Source: CAD feature listing. Evaluate the final solid. Frame: model axes, mm. Face numbers are marked on the shaded views. Give positions to 0.01 mm unless a question says otherwise; leave off trailing zeros. Order: outer loops, then holes, each group sorted by start corner. A loop starts at its lowest first (then second) coordinate and runs counter-clockwise, first axis right, second up.
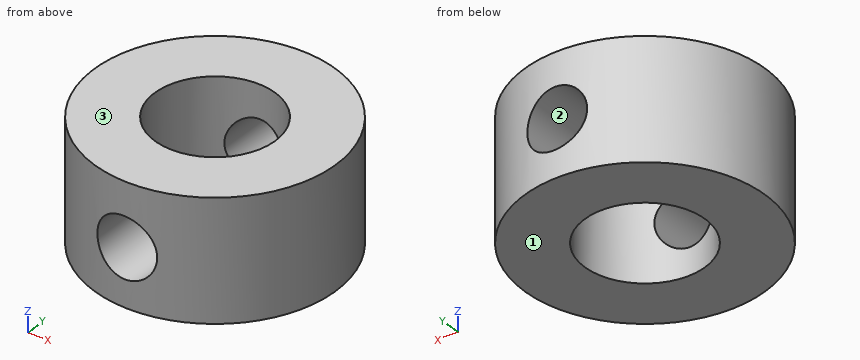
from build123d import *

# Parameters (mm, degrees)
F0_R     = 10
F1_DEPTH = 10
F2_R     = 5
F3_DEPTH = 25
F4_R     = 2.5
F5_DEPTH = 12.5


with BuildPart() as f1:
    # F0 (on Top) → F1 (new body)
    with BuildSketch(Plane.XY):
        Circle(F0_R)
    extrude(amount=F1_DEPTH)

    # F2 (on face) → F3 (cut)
    with BuildSketch(Plane.XY.offset(10)):
        Circle(F2_R)
    extrude(amount=-F3_DEPTH, mode=Mode.SUBTRACT)

    # F4 (on Front) → F5 (cut, symmetric)
    with BuildSketch(Plane.XZ):
        with Locations((0, 4.75)):
            Circle(F4_R)
    extrude(amount=F5_DEPTH, both=True, mode=Mode.SUBTRACT)


solid = f1.part
(1) Section B-B, the plane y = 0. Return loops of the section in (x, z).
(2) Section A-A, the plane x = 0. Return loops of the section in (y, z).
(3) Pin query (flat end, axial travel): pin 1 Ø6 at (x, z) = (0, 4.75) entering from -Y; pin 2 Ø3 at (x, z) = (0, 4.75) entering from -Y; pin 3 Ø1.5 at (x, z) = (-6.5, 5) entering from +Y. Return the tip coordinate at first contact, or that it passes through.
(4) Line query: line 1 along Z through (x, y) = (0, -7); line 2 along Y through (x, z) = (2, 8.5); line 3 along X through (y, z) = (-1, 4). Output: solid intervals per line, ascending.
(5) Section D-D, the plane x = 8.25. Return loops of the section in (y, z).
(6) Draft query along Z for the marked faces 1, 2 and 3. Return one class per face: +Z half, -Z half, draft (parallel to the pull), parting line (faces both ways), or undercut.
(7) Section C-C, the plane z = 5.5. Return loops of the section in (x, y), plus the area to 3 significant figures.
Checks:
1. outline: (-10, 0) - (-5, 0) - (-5, 10) - (-10, 10) - close; (5, 0) - (10, 0) - (10, 10) - (5, 10) - close
2. outline: (-10, 0) - (-5, 0) - (-5, 2.25) - (-10, 2.25) - close; (-10, 7.25) - (-5, 7.25) - (-5, 10) - (-10, 10) - close; (5, 0) - (10, 0) - (10, 2.25) - (5, 2.25) - close; (5, 7.25) - (10, 7.25) - (10, 10) - (5, 10) - close
3. pin 1: stops at y = -10
3. pin 2: passes through
3. pin 3: stops at y = 8.18
4. line 1: z = 0 to 2.25, 7.25 to 10
4. line 2: y = -9.8 to -4.58, 4.58 to 9.8
4. line 3: x = -9.95 to -4.9, 4.9 to 9.95
5. outline: (-5.65, 0) - (5.65, 0) - (5.65, 10) - (-5.65, 10) - close
6. face 1: -Z half
6. face 2: undercut
6. face 3: +Z half
7. outline: (-2.38, -9.71) - (-2.38, -4.39) arc R5 cw to (-2.38, 4.39) - (-2.38, 9.71) arc R10 ccw to start; (2.38, -9.71) arc R10 ccw to (2.38, 9.71) - (2.38, 4.39) arc R5 cw to (2.38, -4.39) - close
7. area: 187 mm2
